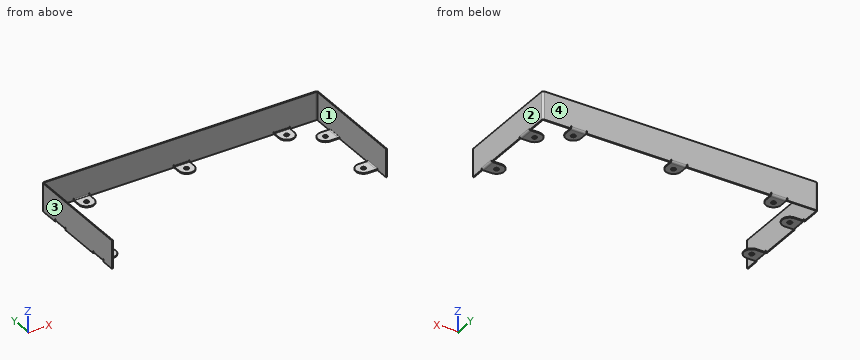
```python
from build123d import *

# Parameters (mm, degrees)
SM_BASE_FLANGE_1_DEPTH            = 28
SM_EDGE_FLANGE_1_STRIP_W          = 6
SM_EDGE_FLANGE_1_STRIP_H          = 1
SM_EDGE_FLANGE_1_STRIP_CUT_DEPTH  = 15.34
SM_EDGE_FLANGE_1_RELIEF_W         = 6.5
SM_EDGE_FLANGE_1_RELIEF_H         = 0.5
SM_EDGE_FLANGE_1_RELIEF_CUT_DEPTH = 1
SM_EDGE_FLANGE_1_DEPTH            = 15.34
SM_EDGE_FLANGE_1_PROFILE_R        = 2.231207153
SM_EDGE_FLANGE_1_FLAT_DEPTH       = 1
PATTERN_LINEAR_1_COUNT            = 2
PATTERN_LINEAR_1_PITCH            = 60
MIRROR_1_COPY_1_SKETCH_W          = 6
MIRROR_1_COPY_1_SKETCH_H          = 1
MIRROR_1_COPY_1_DEPTH             = 15.34
MIRROR_1_COPY_2_SKETCH_W          = 6.5
MIRROR_1_COPY_2_SKETCH_H          = 0.5
MIRROR_1_COPY_2_DEPTH             = 1
MIRROR_1_COPY_3_DEPTH             = 15.34
MIRROR_1_COPY_4_SKETCH_R          = 2.231207153
MIRROR_1_COPY_4_DEPTH             = 1
SM_EDGE_FLANGE_2_STRIP_W          = 6
SM_EDGE_FLANGE_2_STRIP_H          = 1
SM_EDGE_FLANGE_2_STRIP_CUT_DEPTH  = 15.34
SM_EDGE_FLANGE_2_RELIEF_W         = 6.5
SM_EDGE_FLANGE_2_RELIEF_H         = 0.5
SM_EDGE_FLANGE_2_RELIEF_CUT_DEPTH = 1
SM_EDGE_FLANGE_2_DEPTH            = 15.34
SM_EDGE_FLANGE_2_PROFILE_R        = 2.231207153
SM_EDGE_FLANGE_2_FLAT_DEPTH       = 1
PATTERN_LINEAR_2_COUNT            = 3
PATTERN_LINEAR_2_PITCH            = 100


# Sheet-metal steps are written as plain solids
with BuildPart() as part:
    # Sketch 2 → Базовая кромка1 (new body)
    with BuildSketch(Plane.XY):
        with BuildLine():
            Line((-137.5, 0), (-137.5, 108))
            ThreePointArc((-137.5, 108), (-136.914213562, 109.414213562), (-135.5, 110))
            Line((-135.5, 110), (135.5, 110))
            ThreePointArc((135.5, 110), (136.914213562, 109.414213562), (137.5, 108))
            Line((137.5, 108), (137.5, 0))
            Line((137.5, 0), (136.5, 0))
            Line((136.5, 0), (136.5, 108))
            ThreePointArc((136.5, 108), (136.207106781, 108.707106781), (135.5, 109))
            Line((135.5, 109), (-135.5, 109))
            ThreePointArc((-135.5, 109), (-136.207106781, 108.707106781), (-136.5, 108))
            Line((-136.5, 108), (-136.5, 0))
            Line((-136.5, 0), (-137.5, 0))
        make_face()
    extrude(amount=SM_BASE_FLANGE_1_DEPTH)

    # Ребро-кромка1 strip (across the edge) → Ребро-кромка1 strip cut (cut)
    with BuildSketch(Plane(origin=(136.5, 89, 0), x_dir=(0, 0, 1), z_dir=(0, -1, 0))):
        with Locations((-1, -0.5)):
            Rectangle(SM_EDGE_FLANGE_1_STRIP_W, SM_EDGE_FLANGE_1_STRIP_H)
    sm_edge_flange_1_strip_cut = extrude(amount=SM_EDGE_FLANGE_1_STRIP_CUT_DEPTH, mode=Mode.SUBTRACT)

    # Ребро-кромка1 relief (on the sheet) → Ребро-кромка1 relief cut (cut)
    with BuildSketch(Plane(origin=(136.5, 89, 2), x_dir=(0, 0, 1), z_dir=(-1, 0, 0))):
        with Locations((-2.75, 0.25)):
            Rectangle(SM_EDGE_FLANGE_1_RELIEF_W, SM_EDGE_FLANGE_1_RELIEF_H)
        with Locations((-2.75, -15.59)):
            Rectangle(SM_EDGE_FLANGE_1_RELIEF_W, SM_EDGE_FLANGE_1_RELIEF_H)
    sm_edge_flange_1_relief_cut = extrude(amount=-SM_EDGE_FLANGE_1_RELIEF_CUT_DEPTH, mode=Mode.SUBTRACT)

    # Ребро-кромка1 bend section (across the edge) → Ребро-кромка1 (add)
    with BuildSketch(Plane(origin=(136.5, 89, 0), x_dir=(0, 0, 1), z_dir=(0, -1, 0))):
        with BuildLine():
            Line((0, 1), (1, 1))
            ThreePointArc((1, 1), (1.292893219, 0.292893219), (2, 0))
            Line((2, 0), (2, -1))
            ThreePointArc((2, -1), (0.585786438, -0.414213562), (0, 1))
        make_face()
    sm_edge_flange_1 = extrude(amount=SM_EDGE_FLANGE_1_DEPTH)

    # Ребро-кромка1 profile (on flange) → Ребро-кромка1 flat (add)
    with BuildSketch(Plane(origin=(136.5, 0, 0), x_dir=(0, -1, 0), z_dir=(0, 0, -1))):
        with BuildLine():
            ThreePointArc((-73.66, 9), (-81.33, 16.67), (-89, 9))
            Line((-89, 9), (-89, 1))
            Line((-89, 1), (-73.66, 1))
            Line((-73.66, 1), (-73.66, 9))
        make_face()
        with Locations((-81.33, 9)):
            Circle(SM_EDGE_FLANGE_1_PROFILE_R, mode=Mode.SUBTRACT)
    sm_edge_flange_1_flat = extrude(amount=-SM_EDGE_FLANGE_1_FLAT_DEPTH)

    # Линейный массив1: Ребро-кромка1 strip cut, Ребро-кромка1 relief cut, Ребро-кромка1, Ребро-кромка1 flat ×2
    with Locations(*[(0, -i * PATTERN_LINEAR_1_PITCH, 0) for i in range(1, PATTERN_LINEAR_1_COUNT)]):
        add(sm_edge_flange_1_strip_cut, mode=Mode.SUBTRACT)
        add(sm_edge_flange_1_relief_cut, mode=Mode.SUBTRACT)
        add(sm_edge_flange_1)
        add(sm_edge_flange_1_flat)

    # Зеркальное отражение1: Ребро-кромка1 strip cut, Ребро-кромка1 relief cut, Ребро-кромка1, Ребро-кромка1 flat across plane
    add(sm_edge_flange_1_strip_cut.mirror(Plane(origin=(0, 0, 0), x_dir=(0, 0, 1), z_dir=(1, 0, 0))), mode=Mode.SUBTRACT)
    add(sm_edge_flange_1_relief_cut.mirror(Plane(origin=(0, 0, 0), x_dir=(0, 0, 1), z_dir=(1, 0, 0))), mode=Mode.SUBTRACT)
    add(sm_edge_flange_1.mirror(Plane(origin=(0, 0, 0), x_dir=(0, 0, 1), z_dir=(1, 0, 0))))
    add(sm_edge_flange_1_flat.mirror(Plane(origin=(0, 0, 0), x_dir=(0, 0, 1), z_dir=(1, 0, 0))))

    # Зеркальное отражение1 copy 1 sketch → Зеркальное отражение1 copy 1 (cut)
    with BuildSketch(Plane(origin=(-136.5, 29, 0), x_dir=(0, 0, 1), z_dir=(0, -1, 0))):
        with Locations((-1, 0.5)):
            Rectangle(MIRROR_1_COPY_1_SKETCH_W, MIRROR_1_COPY_1_SKETCH_H)
    extrude(amount=MIRROR_1_COPY_1_DEPTH, mode=Mode.SUBTRACT)

    # Зеркальное отражение1 copy 2 sketch → Зеркальное отражение1 copy 2 (cut)
    with BuildSketch(Plane(origin=(-136.5, 29, 2), x_dir=(0, 0, 1), z_dir=(1, 0, 0))):
        with Locations((-2.75, -0.25)):
            Rectangle(MIRROR_1_COPY_2_SKETCH_W, MIRROR_1_COPY_2_SKETCH_H)
        with Locations((-2.75, 15.59)):
            Rectangle(MIRROR_1_COPY_2_SKETCH_W, MIRROR_1_COPY_2_SKETCH_H)
    extrude(amount=-MIRROR_1_COPY_2_DEPTH, mode=Mode.SUBTRACT)

    # Зеркальное отражение1 copy 3 sketch → Зеркальное отражение1 copy 3 (add)
    with BuildSketch(Plane(origin=(-136.5, 29, 0), x_dir=(0, 0, 1), z_dir=(0, -1, 0))):
        with BuildLine():
            Line((0, -1), (1, -1))
            ThreePointArc((1, -1), (1.292893219, -0.292893219), (2, 0))
            Line((2, 0), (2, 1))
            ThreePointArc((2, 1), (0.585786438, 0.414213562), (0, -1))
        make_face()
    extrude(amount=MIRROR_1_COPY_3_DEPTH)

    # Зеркальное отражение1 copy 4 sketch → Зеркальное отражение1 copy 4 (add)
    with BuildSketch(Plane(origin=(-136.5, -60, 0), x_dir=(0, -1, 0), z_dir=(0, 0, -1))):
        with BuildLine():
            ThreePointArc((-73.66, -9), (-81.33, -16.67), (-89, -9))
            Line((-89, -9), (-89, -1))
            Line((-89, -1), (-73.66, -1))
            Line((-73.66, -1), (-73.66, -9))
        make_face()
        with Locations((-81.33, -9)):
            Circle(MIRROR_1_COPY_4_SKETCH_R, mode=Mode.SUBTRACT)
    extrude(amount=-MIRROR_1_COPY_4_DEPTH)

    # Ребро-кромка2 strip (across the edge) → Ребро-кромка2 strip cut (cut)
    with BuildSketch(Plane(origin=(-106.5, 109, 0), x_dir=(0, 0, 1), z_dir=(1, 0, 0))):
        with Locations((-1, -0.5)):
            Rectangle(SM_EDGE_FLANGE_2_STRIP_W, SM_EDGE_FLANGE_2_STRIP_H)
    sm_edge_flange_2_strip_cut = extrude(amount=SM_EDGE_FLANGE_2_STRIP_CUT_DEPTH, mode=Mode.SUBTRACT)

    # Ребро-кромка2 relief (on the sheet) → Ребро-кромка2 relief cut (cut)
    with BuildSketch(Plane(origin=(-106.5, 109, 2), x_dir=(0, 0, 1), z_dir=(0, -1, 0))):
        with Locations((-2.75, 0.25)):
            Rectangle(SM_EDGE_FLANGE_2_RELIEF_W, SM_EDGE_FLANGE_2_RELIEF_H)
        with Locations((-2.75, -15.59)):
            Rectangle(SM_EDGE_FLANGE_2_RELIEF_W, SM_EDGE_FLANGE_2_RELIEF_H)
    sm_edge_flange_2_relief_cut = extrude(amount=-SM_EDGE_FLANGE_2_RELIEF_CUT_DEPTH, mode=Mode.SUBTRACT)

    # Ребро-кромка2 bend section (across the edge) → Ребро-кромка2 (add)
    with BuildSketch(Plane(origin=(-106.5, 109, 0), x_dir=(0, 0, 1), z_dir=(1, 0, 0))):
        with BuildLine():
            Line((0, 1), (1, 1))
            ThreePointArc((1, 1), (1.292893219, 0.292893219), (2, 0))
            Line((2, 0), (2, -1))
            ThreePointArc((2, -1), (0.585786438, -0.414213562), (0, 1))
        make_face()
    sm_edge_flange_2 = extrude(amount=SM_EDGE_FLANGE_2_DEPTH)

    # Ребро-кромка2 profile (on flange) → Ребро-кромка2 flat (add)
    with BuildSketch(Plane(origin=(0, 109, 0), x_dir=(1, 0, 0), z_dir=(0, 0, -1))):
        with BuildLine():
            ThreePointArc((-91.16, 8), (-98.829997184, 15.670005632), (-106.5, 8.000005632))
            Line((-106.5, 8.000005632), (-106.5, 1))
            Line((-106.5, 1), (-91.16, 1))
            Line((-91.16, 1), (-91.16, 8))
        make_face()
        with Locations((-98.83, 8.000005632)):
            Circle(SM_EDGE_FLANGE_2_PROFILE_R, mode=Mode.SUBTRACT)
    sm_edge_flange_2_flat = extrude(amount=-SM_EDGE_FLANGE_2_FLAT_DEPTH)

    # Линейный массив2: Ребро-кромка2 strip cut, Ребро-кромка2 relief cut, Ребро-кромка2, Ребро-кромка2 flat ×3
    with Locations(*[(i * PATTERN_LINEAR_2_PITCH, 0, 0) for i in range(1, PATTERN_LINEAR_2_COUNT)]):
        add(sm_edge_flange_2_strip_cut, mode=Mode.SUBTRACT)
        add(sm_edge_flange_2_relief_cut, mode=Mode.SUBTRACT)
        add(sm_edge_flange_2)
        add(sm_edge_flange_2_flat)


solid = part.part
```
Read the model definition and answer for the solid it produces. Units are mm, in the model's axes. Face numbers are marked on the shaded views. Coordinates: 2 decimals unless noted, no trailing zeros. Write each loop counter-clockwise with the first axis right and the second up, starting at its lowest first coordinate (ties: lowest second). Pieces come first, ordered by that corner, then holes. Notation, with made-up numbers: (42.5, -34) - (95.5, -34) arc R21 cw to (95.5, 5) - close; hole circle Ø11 at (19, 12). An arc over 180 degrees is marked (long way). Answer as a JSON object with one key per item and string values. Group by question number.
1. A cutting plane is placed at A-A (y = 48). Determine the outline of the cut face in (x, z).
2. The mould has two halves that part along X. Classify the marked faces 1, 2, 3 and 4: +X half, -X half, draft (parallel to the pull), parting line (faces both ways), or undercut.
3. A cutting plane is placed at C-C (x = -25.5). Determine the outline of the cut face in (y, z).
4. Consider L1, parallel to Y at x = 127.5, z = 0.6; L2, parallel to X at y = 81.33, z = 0.3; L3, parallel to X at y = 98, z = 15.5. Determine where each line is inside the solid, lowest interval first. Write a range as [from, to].
5. A cutting plane is placed at B-B (z = 19.75). Determine the outline of the cut face in (x, y), plus the area to 3 significant figures.
6. Each of these flat-tipped pins is pushed along its axis until it touches: P1, Ø0.8, axis at x = -132, z = 1.5, coming from the -Y side; P2, Ø2, axis at x = 134, z = 1.5, coming from the -Y side; P3, Ø0.5, axis at y = 109.5, z = 1, coming from the +X side; P4, Ø17, axis at x = 130.5, y = 83, coming from the +Z side. Where does it stop, or does it pass through?
Worked out:
{
 "1": {"outline": "(-137.5, 0) - (-136.5, 0) - (-136.5, 28) - (-137.5, 28) - close; (136.5, 0) - (137.5, 0) - (137.5, 28) - (136.5, 28) - close"},
 "2": {"face 1": "undercut", "face 2": "+X half", "face 3": "-X half", "face 4": "draft"},
 "3": {"outline": "(109, 0) - (110, 0) - (110, 28) - (109, 28) - close"},
 "4": {"L1": "y = [13.66, 19.1], [23.56, 29], [73.66, 79.1], [83.56, 89], [109, 110]", "L2": "x = [-136.55, -129.73], [-125.27, -119.83], [119.83, 125.27], [129.73, 136.55]", "L3": "x = [-137.5, -136.5], [136.5, 137.5]"},
 "5": {"outline": "(-137.5, 0) - (-136.5, 0) - (-136.5, 108) arc R1 cw to (-135.5, 109) - (135.5, 109) arc R1 cw to (136.5, 108) - (136.5, 0) - (137.5, 0) - (137.5, 108) arc R2 ccw to (135.5, 110) - (-135.5, 110) arc R2 ccw to (-137.5, 108) - close", "area": "492 mm²"},
 "6": {"P1": "stops at y = 109", "P2": "stops at y = 13.66", "P3": "stops at x = 137.06", "P4": "stops at z = 28"}
}
